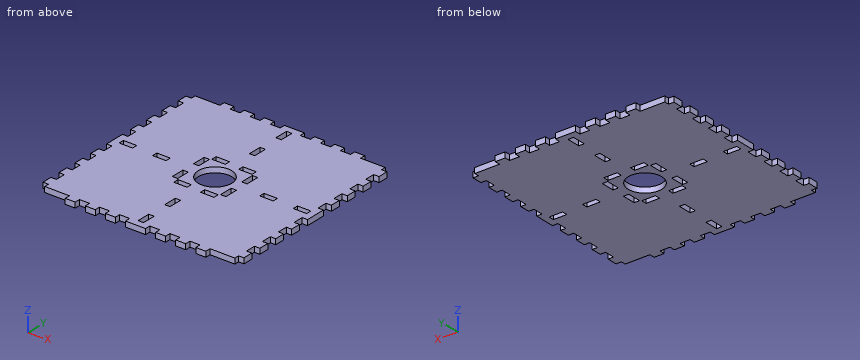
```python
from build123d import *

# Parameters (mm, degrees)
ESQUISSE1_W                  = 300
ESQUISSE1_H                  = 300
BOSS_EXTRU_1_DEPTH           = 8
ESQUISSE3_W                  = 8
ESQUISSE3_H                  = 15
ENL_V_MAT_EXTRU_4_DEPTH      = 213.282830205
ESQUISSE4_R                  = 25
ENL_V_MAT_EXTRU_5_DEPTH      = 213.282830205
ESQUISSE5_W                  = 15
ESQUISSE5_H                  = 8
ESQUISSE5_W_2                = 37
ENL_V_MAT_EXTRU_6_DEPTH      = 213.282830205
ESQUISSE6_W                  = 20
ESQUISSE6_H                  = 8
ENL_V_MAT_EXTRU_7_DEPTH      = 213.282830205
R_P_TITION_CIRCULAIRE1_COUNT = 2
R_P_TITION_CIRCULAIRE1_ANGLE = 90
SYM_TRIE4_COPY_1_SKETCH_W    = 20
SYM_TRIE4_COPY_1_SKETCH_H    = 8
SYM_TRIE4_COPY_1_DEPTH       = 213.282830205
SYM_TRIE4_COPY_2_SKETCH_W    = 20
SYM_TRIE4_COPY_2_SKETCH_H    = 8
SYM_TRIE4_COPY_2_DEPTH       = 213.282830205
ESQUISSE7_W                  = 8
ESQUISSE7_H                  = 20
ENL_V_MAT_EXTRU_8_DEPTH      = 213.282830205
R_P_TITION_CIRCULAIRE2_COUNT = 2
R_P_TITION_CIRCULAIRE2_ANGLE = 90
SYM_TRIE6_COPY_1_SKETCH_W    = 8
SYM_TRIE6_COPY_1_SKETCH_H    = 20
SYM_TRIE6_COPY_1_DEPTH       = 213.282830205
SYM_TRIE6_COPY_2_SKETCH_W    = 8
SYM_TRIE6_COPY_2_SKETCH_H    = 20
SYM_TRIE6_COPY_2_DEPTH       = 213.282830205


with BuildPart() as part:
    # Esquisse1 → Boss.-Extru.1 (new body)
    with BuildSketch(Plane.XY):
        Rectangle(ESQUISSE1_W, ESQUISSE1_H)
    extrude(amount=BOSS_EXTRU_1_DEPTH)

    # Esquisse3 → Enlèv. mat.-Extru.4 (cut, through all)
    with BuildSketch(Plane.XY):
        with Locations((-146, -22.5)):
            Rectangle(ESQUISSE3_W, ESQUISSE3_H)
        with Locations((-146, -52.5)):
            Rectangle(ESQUISSE3_W, ESQUISSE3_H)
        with Locations((-146, -82.5)):
            Rectangle(ESQUISSE3_W, ESQUISSE3_H)
        with Locations((-146, -112.5)):
            Rectangle(ESQUISSE3_W, ESQUISSE3_H)
        with Locations((-146, -142.5)):
            Rectangle(ESQUISSE3_W, ESQUISSE3_H)
        with Locations((-146, 52.5)):
            Rectangle(ESQUISSE3_W, ESQUISSE3_H)
        with Locations((-146, 142.5)):
            Rectangle(ESQUISSE3_W, ESQUISSE3_H)
        with Locations((-146, 112.5)):
            Rectangle(ESQUISSE3_W, ESQUISSE3_H)
        with Locations((-146, 82.5)):
            Rectangle(ESQUISSE3_W, ESQUISSE3_H)
        with Locations((-146, 22.5)):
            Rectangle(ESQUISSE3_W, ESQUISSE3_H)
    enl_v_mat_extru_4 = extrude(amount=ENL_V_MAT_EXTRU_4_DEPTH, mode=Mode.SUBTRACT)

    # Symétrie1: Enlèv. mat.-Extru.4 across plane
    add(enl_v_mat_extru_4.mirror(Plane(origin=(0, 0, 0), x_dir=(0, 0, 1), z_dir=(1, 0, 0))), mode=Mode.SUBTRACT)

    # Esquisse4 → Enlèv. mat.-Extru.5 (cut, through all)
    with BuildSketch(Plane.XY):
        Circle(ESQUISSE4_R)
    extrude(amount=ENL_V_MAT_EXTRU_5_DEPTH, mode=Mode.SUBTRACT)

    # Esquisse5 → Enlèv. mat.-Extru.6 (cut, through all)
    with BuildSketch(Plane.XY):
        with Locations((22.5, 146)):
            Rectangle(ESQUISSE5_W, ESQUISSE5_H)
        with Locations((-22.5, 146)):
            Rectangle(ESQUISSE5_W, ESQUISSE5_H)
        with Locations((-52.5, 146)):
            Rectangle(ESQUISSE5_W, ESQUISSE5_H)
        with Locations((-82.5, 146)):
            Rectangle(ESQUISSE5_W, ESQUISSE5_H)
        with Locations((-123.5, 146)):
            Rectangle(ESQUISSE5_W_2, ESQUISSE5_H)
        with Locations((52.5, 146)):
            Rectangle(ESQUISSE5_W, ESQUISSE5_H)
        with Locations((82.5, 146)):
            Rectangle(ESQUISSE5_W, ESQUISSE5_H)
        with Locations((123.5, 146)):
            Rectangle(ESQUISSE5_W_2, ESQUISSE5_H)
    enl_v_mat_extru_6 = extrude(amount=ENL_V_MAT_EXTRU_6_DEPTH, mode=Mode.SUBTRACT)

    # Symétrie2: Enlèv. mat.-Extru.6 across plane
    add(enl_v_mat_extru_6.mirror(Plane.ZX), mode=Mode.SUBTRACT)

    # Esquisse6 → Enlèv. mat.-Extru.7 (cut, through all)
    with BuildSketch(Plane.XY):
        with Locations((-20, -36)):
            Rectangle(ESQUISSE6_W, ESQUISSE6_H)
        with Locations((20, -36)):
            Rectangle(ESQUISSE6_W, ESQUISSE6_H)
    enl_v_mat_extru_7 = extrude(amount=ENL_V_MAT_EXTRU_7_DEPTH, mode=Mode.SUBTRACT)

    # Symétrie3: Enlèv. mat.-Extru.7 across plane
    add(enl_v_mat_extru_7.mirror(Plane.ZX), mode=Mode.SUBTRACT)

    # Répétition circulaire1: Enlèv. mat.-Extru.7 ×2 about axis
    r_p_tition_circulaire1_axis = Axis((0, 0, 0), (0, 0, 1))
    for i in range(1, R_P_TITION_CIRCULAIRE1_COUNT):
        add(enl_v_mat_extru_7.rotate(r_p_tition_circulaire1_axis, i * R_P_TITION_CIRCULAIRE1_ANGLE / (R_P_TITION_CIRCULAIRE1_COUNT - 1)), mode=Mode.SUBTRACT)

    # Symétrie4 copy 1 sketch → Symétrie4 copy 1 (cut, through all)
    with BuildSketch(Plane(origin=(0, 0, 0), x_dir=(0, 1, 0), z_dir=(0, 0, 1))):
        with Locations((-20, 36)):
            Rectangle(SYM_TRIE4_COPY_1_SKETCH_W, SYM_TRIE4_COPY_1_SKETCH_H)
        with Locations((20, 36)):
            Rectangle(SYM_TRIE4_COPY_1_SKETCH_W, SYM_TRIE4_COPY_1_SKETCH_H)
    extrude(amount=SYM_TRIE4_COPY_1_DEPTH, mode=Mode.SUBTRACT)

    # Symétrie4 copy 2 sketch → Symétrie4 copy 2 (cut, through all)
    with BuildSketch(Plane(origin=(0, 0, 0), x_dir=(-1, 0, 0), z_dir=(0, 0, 1))):
        with Locations((-20, 36)):
            Rectangle(SYM_TRIE4_COPY_2_SKETCH_W, SYM_TRIE4_COPY_2_SKETCH_H)
        with Locations((20, 36)):
            Rectangle(SYM_TRIE4_COPY_2_SKETCH_W, SYM_TRIE4_COPY_2_SKETCH_H)
    extrude(amount=SYM_TRIE4_COPY_2_DEPTH, mode=Mode.SUBTRACT)

    # Esquisse7 → Enlèv. mat.-Extru.8 (cut, through all)
    with BuildSketch(Plane.XY):
        with Locations((0, -130)):
            Rectangle(ESQUISSE7_W, ESQUISSE7_H)
        with Locations((0, -80)):
            Rectangle(ESQUISSE7_W, ESQUISSE7_H)
    enl_v_mat_extru_8 = extrude(amount=ENL_V_MAT_EXTRU_8_DEPTH, mode=Mode.SUBTRACT)

    # Symétrie5: Enlèv. mat.-Extru.8 across plane
    add(enl_v_mat_extru_8.mirror(Plane.ZX), mode=Mode.SUBTRACT)

    # Répétition circulaire2: Enlèv. mat.-Extru.8 ×2 about axis
    r_p_tition_circulaire2_axis = Axis((0, 0, 0), (0, 0, 1))
    for i in range(1, R_P_TITION_CIRCULAIRE2_COUNT):
        add(enl_v_mat_extru_8.rotate(r_p_tition_circulaire2_axis, i * R_P_TITION_CIRCULAIRE2_ANGLE / (R_P_TITION_CIRCULAIRE2_COUNT - 1)), mode=Mode.SUBTRACT)

    # Symétrie6 copy 1 sketch → Symétrie6 copy 1 (cut, through all)
    with BuildSketch(Plane(origin=(0, 0, 0), x_dir=(0, 1, 0), z_dir=(0, 0, 1))):
        with Locations((0, 130)):
            Rectangle(SYM_TRIE6_COPY_1_SKETCH_W, SYM_TRIE6_COPY_1_SKETCH_H)
        with Locations((0, 80)):
            Rectangle(SYM_TRIE6_COPY_1_SKETCH_W, SYM_TRIE6_COPY_1_SKETCH_H)
    extrude(amount=SYM_TRIE6_COPY_1_DEPTH, mode=Mode.SUBTRACT)

    # Symétrie6 copy 2 sketch → Symétrie6 copy 2 (cut, through all)
    with BuildSketch(Plane(origin=(0, 0, 0), x_dir=(-1, 0, 0), z_dir=(0, 0, 1))):
        with Locations((0, 130)):
            Rectangle(SYM_TRIE6_COPY_2_SKETCH_W, SYM_TRIE6_COPY_2_SKETCH_H)
        with Locations((0, 80)):
            Rectangle(SYM_TRIE6_COPY_2_SKETCH_W, SYM_TRIE6_COPY_2_SKETCH_H)
    extrude(amount=SYM_TRIE6_COPY_2_DEPTH, mode=Mode.SUBTRACT)


solid = part.part
```
Could you check a few things on this model? Use its own coordinates, in mm. Round coordinates to 2 decimals unless told otherwise and drop trailing zeros. Loops run counter-clockwise (first coordinate to the right, second up) from the corner with the lowest first, then second, coordinate; pieces in that order, holes last.
Q1. Please list where these lines run through material, in increasing order: L1, parallel to Y at x = 0, z = 5.75; L2, parallel to X at y = -25.5, z = 3.5.
Q2. For P1, Ø2.5, axis at x = 147, z = 3, coming from the -Y side; P2, Ø4, axis at y = 79.5, z = 2, coming from the +X side; P3, Ø4, axis at y = 146, z = 5.5, coming from the -X side, each with a flat end and sliding along its axis, tell me the tip position at first contact or that it passes through.
Q3. I want a section at B-B (x = 126). Write out the boundary of the cut face in (y, z).
Q4. I want a section at A-A (y = 0). Write out the boundary of the cut face in (x, z).
Answer below:
1. L1: y = -150 to -140, -120 to -90, -70 to -25, 25 to 70, 90 to 120, 140 to 150
1. L2: x = -142 to -40, -32 to 32, 40 to 142
2. P1: stops at y = -135
2. P2: stops at x = 142
2. P3: stops at x = -105
3. outline: (-142, 0) - (-4, 0) - (-4, 8) - (-142, 8) - close; (4, 0) - (142, 0) - (142, 8) - (4, 8) - close
4. outline: (-150, 0) - (-140, 0) - (-140, 8) - (-150, 8) - close; (-120, 0) - (-90, 0) - (-90, 8) - (-120, 8) - close; (-70, 0) - (-25, 0) - (-25, 8) - (-70, 8) - close; (25, 0) - (70, 0) - (70, 8) - (25, 8) - close; (90, 0) - (120, 0) - (120, 8) - (90, 8) - close; (140, 0) - (150, 0) - (150, 8) - (140, 8) - close
